from build123d import *

# Parameters (mm, degrees)
SKETCH1_W           = 38.1
SKETCH1_H           = 23.114
BOSS_EXTRUDE1_DEPTH = 5.334
SKETCH2_W           = 22.86
SKETCH2_H           = 21.9964
BOSS_EXTRUDE2_DEPTH = 2.8956
SKETCH3_W           = 7.4422
SKETCH3_H           = 3.6576
BOSS_EXTRUDE3_DEPTH = 4.7498
SKETCH4_W           = 6.6802
SKETCH4_H           = 2.8956
CUT_EXTRUDE1_DEPTH  = 3.556
SKETCH5_W           = 5.9182
SKETCH5_H           = 3.6576
BOSS_EXTRUDE4_DEPTH = 1.651
SKETCH6_W           = 5.1562
SKETCH6_H           = 2.8956
CUT_EXTRUDE2_DEPTH  = 3.3782
LPATTERN1_COUNT     = 3
LPATTERN1_PITCH     = 5.969


with BuildPart() as part:
    # Sketch1 → Boss-Extrude1 (new body)
    with BuildSketch(Plane(origin=(0, 0, 0), x_dir=(1, 0, 0), z_dir=(0, 1, 0))):
        with Locations((19.05, 11.557)):
            Rectangle(SKETCH1_W, SKETCH1_H)
    extrude(amount=BOSS_EXTRUDE1_DEPTH)

    # Sketch2 → Boss-Extrude2 (add)
    with BuildSketch(Plane(origin=(0, 5.334, 0), x_dir=(1, 0, 0), z_dir=(0, 1, 0))):
        with Locations((16.4338, 11.557)):
            Rectangle(SKETCH2_W, SKETCH2_H)
    extrude(amount=BOSS_EXTRUDE2_DEPTH)

    # Sketch3 → Boss-Extrude3 (add)
    with BuildSketch(Plane.XY):
        with Locations((28.2829, 2.667)):
            Rectangle(SKETCH3_W, SKETCH3_H)
    extrude(amount=BOSS_EXTRUDE3_DEPTH)

    # Sketch4 → Cut-Extrude1 (cut)
    with BuildSketch(Plane.XY.offset(4.7498)):
        with Locations((28.2829, 2.667)):
            Rectangle(SKETCH4_W, SKETCH4_H)
    extrude(amount=-CUT_EXTRUDE1_DEPTH, mode=Mode.SUBTRACT)

    # Sketch5 → Boss-Extrude4 (add)
    with BuildSketch(Plane(origin=(38.1, 0, 0), x_dir=(0, 0, -1), z_dir=(1, 0, 0))):
        with Locations((5.4991, 2.667)):
            Rectangle(SKETCH5_W, SKETCH5_H)
    boss_extrude4 = extrude(amount=BOSS_EXTRUDE4_DEPTH)

    # Sketch6 → Cut-Extrude2 (cut)
    with BuildSketch(Plane(origin=(39.751, 0, 0), x_dir=(0, 0, -1), z_dir=(1, 0, 0))):
        with Locations((5.4991, 2.667)):
            Rectangle(SKETCH6_W, SKETCH6_H)
    cut_extrude2 = extrude(amount=-CUT_EXTRUDE2_DEPTH, mode=Mode.SUBTRACT)

    # LPattern1: Boss-Extrude4, Cut-Extrude2 ×3
    with Locations(*[(0, 0, -i * LPATTERN1_PITCH) for i in range(1, LPATTERN1_COUNT)]):
        add(boss_extrude4)
        add(cut_extrude2, mode=Mode.SUBTRACT)


solid = part.part
Work out the finished part from the listing and answer in its coordinate system (mm). A direction names the side the tool comes from. Give positions to 0.01 mm unless a question says otherwise; leave off trailing zeros. Order: outer loops, then holes, each group sorted by start corner. A loop starts at its lowest first (then second) coordinate and runs counter-clockwise, first axis right, second up. Notation, with made-up numbers: (-26.75, -19.5) - (-21.75, -19.5) arc R18 ccw to (-21.75, 11.5) - close; hole circle Ø7 at (46.5, -19.75). An arc over 180 degrees is marked (long way). Answer as CSV lines item,"result". Start each with the question number.
Q1. The mould has two halves that part along Z. Classify faces 4 (the face through (19, 3, -23.114)), 5 (the face through (36.373, 3, -17)), 6 (the face through (39, 0.838, -17)): +Z half, -Z half, draft (parallel to the pull), parting line (faces both ways), or undercut.
Q2. The part is cut by section B-B (z = 2.25). Write down the section's boundary in (x, y), then the cut area to 3 significant figures.
Q3. For faces 1 (the face through (39, 3, -2.54)), 2 (the face through (38, 1.219, -17)), 3 (the face through (28, 0.838, 2)), determine the directions among +Z, -Z, +X, -X, +Y, -Y from which every point of the face is accessible in a straight line to the end or side of a thin tool.
Q4. The part is cut by section D-D (z = -5.75). Write down the section's boundary in (x, y).
Q5. The part is cut by section A-A (x = 29.5). Write down the section's boundary in (y, z), then the cut area to 3 significant figures.
Q6. The part is cut by section C-C (y = 5.75). Write down the section's boundary in (x, z), then the cut area to 3 significant figures.
Q7. Given pin 1 Ø1.4 at (x, z) = (28, 3) entering from -Y; pin 2 Ø2.5 at (y, z) = (2.5, -5.5) entering from +X; pin 3 Ø0.9 at (x, y) = (26.5, 2) entering from +Z, each flat-ended and moving along its own axis, determine where each tip first touches the part or whether it passes through.
Q8. Find the intervals of material crossed by L1, parallel to Z at x = 26, y = 5; L2, parallel to X at y = 1.5, z = 1.25; L3, parallel to Y at x = 33, z = -4.25, in increasing order. Write a range as [from, to].
Check result:
1,face 4,"-Z half"
1,face 5,"undercut"
1,face 6,"draft"
2,outline,"(24.56, 0.84) - (32, 0.84) - (32, 4.5) - (24.56, 4.5) - close; hole (24.94, 1.22) - (31.62, 1.22) - (31.62, 4.11) - (24.94, 4.11) - close"
2,area,"7.88 mm²"
3,face 1,"+Z, +X, +Y, -Y"
3,face 2,"+X"
3,face 3,"+Z, +X, -X, -Y"
4,outline,"(0, 0) - (38.1, 0) - (38.1, 0.84) - (39.75, 0.84) - (39.75, 1.22) - (36.37, 1.22) - (36.37, 4.11) - (39.75, 4.11) - (39.75, 4.5) - (38.1, 4.5) - (38.1, 5.33) - (27.86, 5.33) - (27.86, 8.23) - (5, 8.23) - (5, 5.33) - (0, 5.33) - close"
5,outline,"(0, -23.11) - (5.33, -23.11) - (5.33, 0) - (4.5, 0) - (4.5, 4.75) - (4.11, 4.75) - (4.11, 1.19) - (1.22, 1.19) - (1.22, 4.75) - (0.84, 4.75) - (0.84, 0) - (0, 0) - close"
5,area,"130 mm²"
6,outline,"(5, -22.56) - (27.86, -22.56) - (27.86, -0.56) - (5, -0.56) - close"
6,area,"503 mm²"
7,pin 1,"stops at y = 0.84"
7,pin 2,"stops at x = 36.37"
7,pin 3,"stops at z = 1.19"
8,L1,"z = [-23.11, 0]"
8,L2,"x = [24.56, 24.94], [31.62, 32]"
8,L3,"y = [0, 5.33]"
